Work out the finished part from the listing and answer in its coordinate system (mm). Face numbers are marked on the shaded views. Round coordinates to 2 decimals unless told otherwise and drop trailing zeros. Write each loop counter-clockwise with the first axis right and the second up, starting at its lowest first coordinate (ties: lowest second). Pieces come first, ordered by that corner, then holes. Notation, with made-up numbers: M 22,78 L 49,78 A25 ccw 49,108 Z; hole C 61,36.25 d8. An arc over 180 degrees is marked long. Answer in a Markdown table with one row per item.
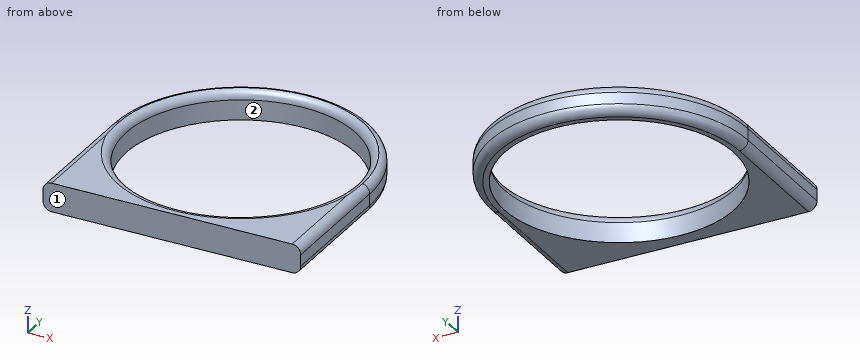
```python
from build123d import *

# Parameters (mm, degrees)
F1_DEPTH    = 10
F2_T1_DEPTH = 52.5
F2_T6_ANGLE = 180
F2_T8_ANGLE = 180


# Not quite as in the source:
# - a fillet or chamfer that OpenCascade refuses, or shapes differently, is made with other operations: its cross-section is extruded or revolved along the edge and cut away or added


with BuildPart() as f1:
    # F0 (on Top) → F1 (new body)
    with BuildSketch(Plane.XY):
        with BuildLine():
            Line((45, -45), (45, 0))
            ThreePointArc((45, 0), (0, 45), (-45, 0))
            Line((-45, 0), (-45, -45))
            Line((-45, -45), (0, -45))
            Line((0, -45), (45, -45))
        make_face()
        with BuildLine():
            ThreePointArc((0, 40), (40, 0), (0, -40))
            ThreePointArc((0, -40), (-40, 0), (0, 40))
        make_face(mode=Mode.SUBTRACT)
    extrude(amount=F1_DEPTH)

    # F2: fillet of radius 3 on 6 edges, made by hand

    # F2_s2 → F2_t1 (cut)
    with BuildSketch(Plane.XZ):
        with BuildLine():
            ThreePointArc((-42, 10), (-44.1213203436, 9.1213203436), (-45, 7))
            Line((-45, 7), (-45, 10))
            Line((-45, 10), (-42, 10))
        make_face()
        with BuildLine():
            ThreePointArc((-45, 3), (-44.1213203436, 0.8786796564), (-42, 0))
            Line((-42, 0), (-45, 0))
            Line((-45, 0), (-45, 3))
        make_face()
        with BuildLine():
            ThreePointArc((45, 3), (44.1213203436, 0.8786796564), (42, 0))
            Line((42, 0), (45, 0))
            Line((45, 0), (45, 3))
        make_face()
        with BuildLine():
            ThreePointArc((45, 7), (44.1213203436, 9.1213203436), (42, 10))
            Line((42, 10), (45, 10))
            Line((45, 10), (45, 7))
        make_face()
    extrude(amount=F2_T1_DEPTH, mode=Mode.SUBTRACT)

    # F2_s3 → F2_t4 (revolve, cut)
    with BuildSketch(Plane.YZ):
        with BuildLine():
            ThreePointArc((43, 10), (40.8786796564, 9.1213203436), (40, 7))
            Line((40, 7), (40, 10))
            Line((40, 10), (43, 10))
        make_face()
    revolve(axis=Axis((0, 0, 10), (0, 0, 1)), mode=Mode.SUBTRACT)

    # F2_s5 → F2_t6 (revolve, cut)
    with BuildSketch(Plane.XZ):
        with BuildLine():
            ThreePointArc((42, 10), (44.1213203436, 9.1213203436), (45, 7))
            Line((45, 7), (45, 10))
            Line((45, 10), (42, 10))
        make_face()
    revolve(axis=Axis((0, 0, 10), (0, 0, 1)), revolution_arc=F2_T6_ANGLE, mode=Mode.SUBTRACT)

    # F2_s7 → F2_t8 (revolve, cut)
    with BuildSketch(Plane.XZ):
        with BuildLine():
            ThreePointArc((42, 0), (44.1213203436, 0.8786796564), (45, 3))
            Line((45, 3), (45, 0))
            Line((45, 0), (42, 0))
        make_face()
    revolve(axis=Axis((0, 0, 0), (0, 0, 1)), revolution_arc=F2_T8_ANGLE, mode=Mode.SUBTRACT)


solid = f1.part
```
1. Consider line 1 along X through (y, z) = (10, 5.5); line 2 along X through (y, z) = (0, 3.25); line 3 along Y through (x, z) = (-28, 4). Determine where each line is inside the solid, lowest interval first. Write a range as from..to.
Calculated:
| item | result |
|---|---|
| line 1 | x = -43.87..-38.73, 38.73..43.87 |
| line 2 | x = -45..-40, 40..45 |
| line 3 | y = -45..-28.57, 28.57..35.23 |
2. Determine the mould class of the marked faces 1 and 2 for opening direction X: released by +X, released by -X, zero draft, split by the parting line, or undercut.
Calculated:
| item | result |
|---|---|
| face 1 | zero draft |
| face 2 | undercut |
3. The part is cut by section A-A (x = 0). Determine the outline of the cut face in (y, z).
Calculated:
| item | result |
|---|---|
| outline | M -45,0 L -40,0 L -40,7 A3 ccw -43,10 L -45,10 Z; M 40,0 L 42,0 A3 ccw 45,3 L 45,7 A3 ccw 42.5,9.96 A3 ccw 40,7 Z |
4. Given pin 1 (4 mm diameter, centred on y = 33.5, z = 9, fed in from +X); pin 2 (1.5 mm diameter, centred on x = 32.5, y = 29, fed in from +Z); pin 3 (2 mm diameter, centred on y = 22.5, z = 4, fed in from +X), each flat-ended and moving along its own axis, determine where each tip first touches the part or whether it passes through.
Calculated:
| item | result |
|---|---|
| pin 1 | stops at x = 31.63 |
| pin 2 | stops at z = 9.89 |
| pin 3 | stops at x = 39.53 |
